Input: part model. Units: mm. Frame: model coordinates. Round coordinates to 2 decimals unless told otherwise and drop trailing zeros.
1) Ray query, line 1 along Y through (x, z) = (265, 2.4); line 2 along X through (y, z) = (-190, 2.05); line 3 along Y through (x, z) = (-145, 2.25). Return the intervals inside material, ascending.
2) Section A-A, the plane z = 1.55. State how many separate pieces and enclosed holes the cut face has, and give its area (3 significant figures).
3) First-contact query: pin 1 (1.5 mm diameter, centred on x = 238, z = 1.5, fed in from +Y); pin 2 (1.5 mm diameter, centred on y = 246, z = 2.5, fed in from -X); pin 3 (1.5 mm diameter, centred on x = -144.5, z = 3.5, fed in from +Y). Flat tips, straight axial feed; report the tip coordinate or a pass-through.
from build123d import *

# Parameters (mm, degrees)
SKETCH_1_W          = 550
SKETCH_1_H          = 520
EXTRUDE_1_DEPTH     = 5
SKETCH_2_R          = 2.5
CUT_EXTRUDE_1_DEPTH = 379.483817356
FILLET_1_R          = 5


with BuildPart() as part:
    # 草图1 → 凸台-拉伸1 (new body)
    with BuildSketch(Plane.XY):
        Rectangle(SKETCH_1_W, SKETCH_1_H)
    extrude(amount=EXTRUDE_1_DEPTH)

    # 草图2 → 切除-拉伸1 (cut, through all)
    with BuildSketch(Plane.XY.offset(5)):
        with Locations((205, 250)):
            Circle(SKETCH_2_R)
        with Locations((265, 190)):
            Circle(SKETCH_2_R)
        with Locations((-265, -190)):
            Circle(SKETCH_2_R)
        with Locations((205, -250)):
            Circle(SKETCH_2_R)
        with Locations((265, -190)):
            Circle(SKETCH_2_R)
        with Locations(Location((-265, 190, 0), (0, 0, 180))):
            Circle(SKETCH_2_R)
        with Locations((-115, 250)):
            Circle(SKETCH_2_R)
        with Locations((-115, -250)):
            Circle(SKETCH_2_R)
        with Locations((-145, -195)):
            Circle(SKETCH_2_R)
        with Locations((-145, 195)):
            Circle(SKETCH_2_R)
        Polygon((255, 240), (215, 240), (215, 260), (275, 260), (275, 200), (255, 200), align=None)
        Polygon((-255, -240), (-155, -240), (-155, -215), (-135, -215), (-135, -260), (-275, -260), (-275, -200), (-255, -200), align=None)
        Polygon((255, -240), (255, -200), (275, -200), (275, -260), (215, -260), (215, -240), align=None)
        Polygon((-275, 260), (-135, 260), (-135, 215), (-155, 215), (-155, 240), (-255, 240), (-255, 200), (-275, 200), align=None)
    extrude(amount=-CUT_EXTRUDE_1_DEPTH, mode=Mode.SUBTRACT)

    # 圆角1
    fillet_1_edges = [part.edges().sort_by_distance(p)[0] for p in [
        (215, -260, 2.5),
        (215, -240, 2.5),
        (255, -240, 2.5),
        (255, -200, 2.5),
        (275, -200, 2.5),
        (275, 200, 2.5),
        (255, 200, 2.5),
        (255, 240, 2.5),
        (215, 240, 2.5),
        (215, 260, 2.5),
        (-275, 200, 2.5),
        (-135, 260, 2.5),
        (-135, 215, 2.5),
        (-155, 215, 2.5),
        (-155, 240, 2.5),
        (-255, 240, 2.5),
        (-255, 200, 2.5),
        (-275, -200, 2.5),
        (-255, -200, 2.5),
        (-255, -240, 2.5),
        (-155, -240, 2.5),
        (-155, -215, 2.5),
        (-135, -215, 2.5),
        (-135, -260, 2.5),
    ]]
    fillet(fillet_1_edges, radius=FILLET_1_R)


solid = part.part
Final values:
1. line 1: y = -200 to -192.5, -187.5 to 187.5, 192.5 to 200
1. line 2: x = -275 to -267.5, -262.5 to 262.5, 267.5 to 275
1. line 3: y = -215 to -197.5, -192.5 to 192.5, 197.5 to 215
2. separate pieces: 1
2. enclosed holes: 10
2. area: 274,000 mm2
3. pin 1: stops at y = 240
3. pin 2: stops at x = -135
3. pin 3: stops at y = 215
